Source: CAD feature listing. Evaluate the final solid. Frame: model axes, mm. A direction names the side the tool comes from. Round coordinates to 2 decimals unless told otherwise and drop trailing zeros. Write each loop counter-clockwise with the first axis right and the second up, starting at its lowest first coordinate (ties: lowest second). Pieces come first, ordered by that corner, then holes. Notation, with made-up numbers: M -1,-7.5 L 47,-7.5 A16 cw 47,10.5 Z; hole C 41,-32.5 d10. An arc over 180 degrees is marked long. Answer in a Markdown table with one row per item. Add a question column.
Item 1: Set-up query: faces 1 (the face through (0, 7, 0)), 2 (the face through (-2.3, 1, 0.1)), 3 (the face through (0.601, 3.465, 1.908)). Return all of +Z, -Z, +X, -X, +Y, -Y with unobstructed straight access to the full face (end or side cutting, diameter ignored); none if empty.
Item 2: Mould query, pull axis Y, two halves, no side actions, for faces 4 (the face through (0, 6, 0)), 5 (the face through (0, 1.5, 3)), 6 (the face through (0, 0, 0)). Classes: released by +Y, released by -Y, zero draft, split by the parting line, or undercut.
Item 3: Contact query for flat-ended pins moving along their axis: pin 1 (4 mm diameter, centred on x = -2, y = 6, fed in from -Z); pin 2 (0.9 mm diameter, centred on x = 0.5, z = 3, fed in from +Y); pin 3 (2 mm diameter, centred on x = -1.5, y = 6.5, fed in from -Z). Output: stop coordinate, or through.
Item 4: Cut plane B-B on x = 0. Return loops of the section in (y, z).
Item 5: Cut plane C-C on y = 1.25. Return loops of the section in (x, z), and give its area (3 significant figures).
Item 6: Cut plane A-A on z = 0. Return loops of the section in (x, y).
Item 7: Material intervals for probe 1 along Y at (x, z) = (-1.25, 2.5); probe 2 along Z at (x, y) = (0.5, 4.25); probe 3 along X at (y, z) = (5, -0.25), sorted ascending.
Item 8: Cut plane D-D on z = -3. Return loops of the section in (x, y), and give its area (3 significant figures).
from build123d import *

# Parameters (mm, degrees)
SKETCH2_R           = 3.45
BOSS_EXTRUDE1_DEPTH = 1
SKETCH4_R           = 2
BOSS_EXTRUDE2_DEPTH = 5
CUT_EXTRUDE1_DEPTH  = 0.5
BOSS_EXTRUDE3_DEPTH = 0.5


with BuildPart() as part:
    # Sketch2 → Boss-Extrude1 (new body)
    with BuildSketch(Plane(origin=(0, 0, 0), x_dir=(1, 0, 0), z_dir=(0, 1, 0))):
        with Locations(Location((0, 0, 0), (0, 0, 270))):
            Circle(SKETCH2_R)
    extrude(amount=BOSS_EXTRUDE1_DEPTH)

    # Sketch4 → Boss-Extrude2 (add)
    with BuildSketch(Plane(origin=(0, 1, 0), x_dir=(1, 0, 0), z_dir=(0, 1, 0))):
        with Locations(Location((0, 0, 0), (0, 0, 270))):
            Circle(SKETCH4_R)
    extrude(amount=BOSS_EXTRUDE2_DEPTH)

    # Sketch5 → Revolve1 (revolve)
    with BuildSketch(Plane(origin=(0, 0, 0), x_dir=(0, 0, -1), z_dir=(1, 0, 0)), mode=Mode.PRIVATE) as revolve1_sk:
        with BuildLine():
            Line((0, 0), (-1, 0))
            Line((-1, 0), (-2, 6))
            ThreePointArc((-2, 6), (-1.414213562, 7.414213562), (0, 8))
            Line((0, 8), (0, 0))
        make_face()
    revolve(revolve1_sk.sketch.rotate(Axis((0, 0, 0), (0, 1, 0)), 180), axis=Axis((0, 0, 0), (0, 1, 0)))

    # Sketch8 → Cut-Extrude1 (cut, symmetric)
    with BuildSketch(Plane.XY):
        with BuildLine():
            Line((-2, 4), (-2, 7))
            Line((-2, 7), (2, 7))
            Line((2, 7), (2, 4))
            ThreePointArc((2, 4), (0, 6), (-2, 4))
        make_face()
    extrude(amount=CUT_EXTRUDE1_DEPTH, both=True, mode=Mode.SUBTRACT)

    # Sketch10 → Boss-Extrude3 (add)
    with BuildSketch(Plane(origin=(0, 1, 0), x_dir=(1, 0, 0), z_dir=(0, 1, 0))):
        with BuildLine():
            Line((-1.431879851, 3.138824635), (-0.55021537, -3.405842487))
            ThreePointArc((-0.55021537, -3.405842487), (0.460605794, -3.419114257), (1.431879851, -3.138824635))
            Line((1.431879851, -3.138824635), (0.55021537, 3.405842487))
            ThreePointArc((0.55021537, 3.405842487), (-0.460605794, 3.419114257), (-1.431879851, 3.138824635))
        make_face()
    extrude(amount=BOSS_EXTRUDE3_DEPTH)


solid = part.part
Results below:
| question | item | result |
|---|---|---|
| 1 | face 1 | +X, -X |
| 1 | face 2 | -X, +Y |
| 1 | face 3 | +Y |
| 2 | face 4 | undercut |
| 2 | face 5 | released by +Y |
| 2 | face 6 | released by -Y |
| 3 | pin 1 | z = -2 |
| 3 | pin 2 | y = 1.5 |
| 3 | pin 3 | z = -1.91 |
| 4 | outline | M 0,-3.45 L 1.5,-3.45 L 1.5,-2 L 6,-2 A2 ccw 6,2 L 1.5,2 L 1.5,3.45 L 0,3.45 Z; hole M 6,-0.5 L 7,-0.5 L 7,0.5 L 6,0.5 Z |
| 5 | outline | M -1.43,-3.14 A3.45 ccw 0.55,-3.41 L 0.76,-1.85 A2 ccw 1.22,1.58 L 1.43,3.14 A3.45 ccw -0.55,3.41 L -0.76,1.85 A2 ccw -1.22,-1.58 Z |
| 5 | area | 18.5 mm2 |
| 6 | outline | M -3.45,0 L 3.45,0 L 3.45,1 L 2,1 L 2,4 A2 ccw -2,4 L -2,1 L -3.45,1 Z; M -1.73,7 L 1.73,7 A2 ccw Z |
| 7 | probe 1 | 0 to 1 |
| 7 | probe 2 | -1.94 to 1.94 |
| 7 | probe 3 | -1.73 to 1.73 |
| 8 | outline | M -1.7,0 L 1.7,0 L 1.7,1 L 0.6,1 L 0.6,1.5 L -1.41,1.5 L -1.41,1 L -1.7,1 Z |
| 8 | area | 4.42 mm2 |
